Design review of the part shown in the three views and the two pictorial views. Dimensions are in mm from the part's minimum x, y and z. Give positions to 0.01 mm unless a question says otherwise; leave off trailing zeros. Loops run counter-clockwise (first coordinate to the right, second up) from the corner with the lowest first, then second, coordinate; pieces in that order, holes last. Notation, with made-up numbers: (39, -12) -> (58, -12) arc R19 ccw to (58, 1) -> close; hole circle Ø1 at (6.5, 48.25). An arc over 180 degrees is marked (long way). One line per question, with ' | ' between items. Start each with the question number.
(1) Consider section C-C (y = 47). Write out the cut boundary in (x, z), and give its area (3 significant figures).
(2) Consider section A-A (x = 31.75). Write out the cut boundary in (y, z) (3 decimals).
(3) Consider section B-B (z = 31.75). Write out the cut boundary in (x, y) (3 decimals), and give its area (3 significant figures).
(4) Wall thickness on probe 1 along Z at (x, y) = (31.75, 27); probe 2 along X at (y, z) = (44.5, 28): over which ranges is each line inside the solid? List them lowest first.
(5) Draft analysis for pull direction Z (two halves, no side actions). For the marked faces 1, 2 and 3, state which applies: +Z half, -Z half, draft (parallel to the pull), parting line (faces both ways), or undercut.
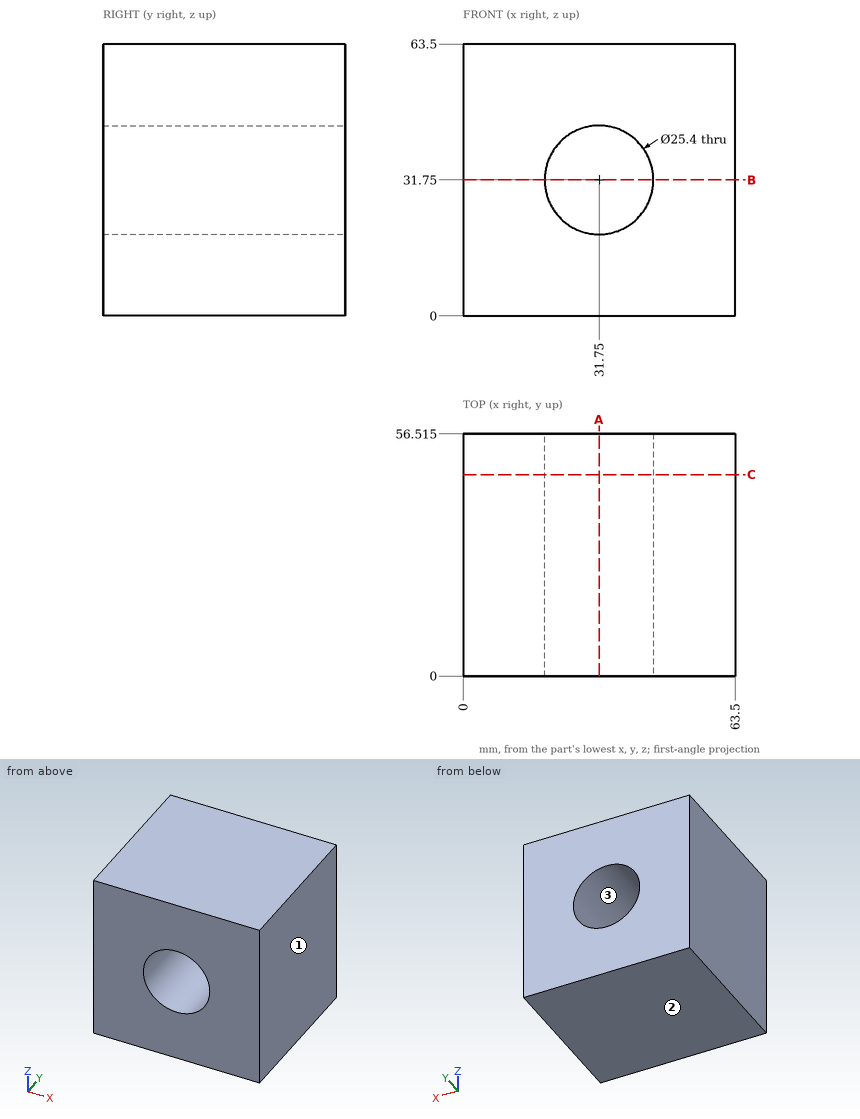
A:
1) outline: (0, 0) -> (63.5, 0) -> (63.5, 63.5) -> (0, 63.5) -> close; hole circle Ø25.4 at (31.75, 31.75) | area: 3,530 mm^2
2) outline: (0, 0) -> (56.515, 0) -> (56.515, 19.05) -> (0, 19.05) -> close; (0, 44.45) -> (56.515, 44.45) -> (56.515, 63.5) -> (0, 63.5) -> close
3) outline: (0, 0) -> (19.05, 0) -> (19.05, 56.515) -> (0, 56.515) -> close; (44.45, 0) -> (63.5, 0) -> (63.5, 56.515) -> (44.45, 56.515) -> close | area: 2,150 mm^2
4) probe 1: z = 0 to 19.05, 44.45 to 63.5 | probe 2: x = 0 to 19.62, 43.88 to 63.5
5) face 1: draft | face 2: -Z half | face 3: undercut
